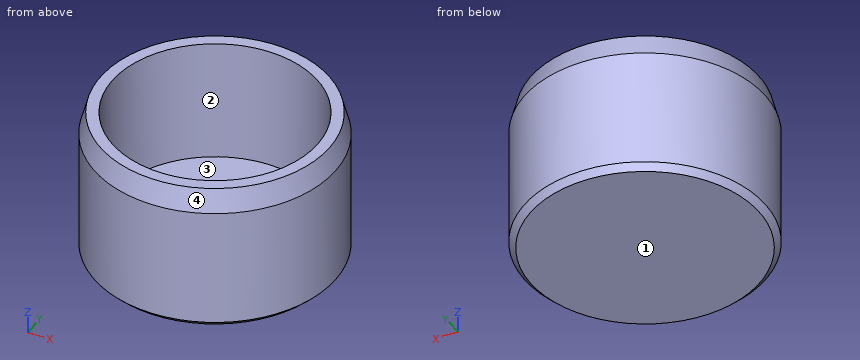
from build123d import *

# Parameters (mm, degrees)
F0_R     = 24.765
F0_R_2   = 21.082
F1_DEPTH = 30.48
F2_DEPTH = 5.08
F3_SIZE2 = 4.7397045256
F3_SIZE  = 1.27
F4_SIZE  = 1.27


with BuildPart() as f1:
    # F0 (on Top) → F1 (new body)
    with BuildSketch(Plane.XY):
        Circle(F0_R)
        Circle(F0_R_2, mode=Mode.SUBTRACT)
    extrude(amount=F1_DEPTH)

    # F0 (on Top) → F2 (join)
    with BuildSketch(Plane.XY):
        Circle(F0_R)
        Circle(F0_R_2, mode=Mode.SUBTRACT)
        Circle(F0_R_2)
    extrude(amount=F2_DEPTH)

    # F3
    f3_edges = [f1.edges().sort_by_distance(p)[0] for p in [
        (-24.765, 0, 30.48),
    ]]
    f3_side = f1.faces().sort_by_distance((-24.06454, 0, 30.48))[0]
    chamfer(f3_edges, length=F3_SIZE, length2=F3_SIZE2, reference=f3_side)

    # F4
    f4_edges = [f1.edges().sort_by_distance(p)[0] for p in [
        (-24.765, 0, 0),
    ]]
    chamfer(f4_edges, length=F4_SIZE)


solid = f1.part
Design review of the part built by this model. Coordinates are the model's own, in mm. Face numbers are marked on the shaded views. Round coordinates to 2 decimals unless told otherwise and drop trailing zeros. Write each loop counter-clockwise with the first axis right and the second up, starting at its lowest first coordinate (ties: lowest second). Pieces come first, ordered by that corner, then holes. Notation, with made-up numbers: (-19, 56.5) - (15, 56.5) arc R25 ccw to (15, 81.5) - close; hole circle Ø11 at (-31.5, 84.5). An arc over 180 degrees is marked (long way). Return JSON: item names as keys, results as strings. Group by question number.
Item 1: For probe 1 along Y at (x, z) = (0, 12.5) (3 decimals); probe 2 along Z at (x, y) = (17, -5.5); probe 3 along X at (y, z) = (0.5, 19), list the stretches that pass through material, from the lowest coordinate up. Write a range as [from, to].
Item 2: The part is to be moulded in two halves that separate along Y. For the marked faces 1, 2, 3 and 4, say which applies: pulls with the +Y half, pulls with the -Y half, needs draft (parallel to the pull), parting line crosses it, or undercut.
Item 3: We need section D-D on z = 4. Write out the cut boundary in (x, y) (3 decimals).
Item 4: We need section C-C on z = 13.5. Write out the cut boundary in (x, y) (3 decimals).
Item 5: We need section A-A on y = 0. Write out the cut boundary in (x, z) (3 decimals), and give its area (3 significant figures).
Item 6: Insertion check: P1, Ø8, axis at y = -5, z = 17.5, coming from the -X side; P2, Ø1, axis at x = -15.5, y = 12.5, coming from the +Z side; P3, Ø4, axis at y = -6, z = 3, coming from the -X side; P4, Ø5, axis at x = -8.5, y = 6.5, coming from the -Z side. Each pin has a flat end and moves straight along its axis. Give the tip position at first contact, or say it passes through.
Model answer:
{
 "1": {"probe 1": "y = [-24.765, -21.082], [21.082, 24.765]", "probe 2": "z = [0, 5.08]", "probe 3": "x = [-24.76, -21.08], [21.08, 24.76]"},
 "2": {"face 1": "needs draft", "face 2": "undercut", "face 3": "undercut", "face 4": "parting line crosses it"},
 "3": {"outline": "circle Ø49.53 at (0, 0)"},
 "4": {"outline": "circle Ø49.53 at (0, 0); hole circle Ø42.164 at (0, 0)"},
 "5": {"outline": "(-24.765, 1.27) - (-23.495, 0) - (23.495, 0) - (24.765, 1.27) - (24.765, 25.74) - (23.495, 30.48) - (21.082, 30.48) - (21.082, 5.08) - (-21.082, 5.08) - (-21.082, 30.48) - (-23.495, 30.48) - (-24.765, 25.74) - close", "area": "431 mm²"},
 "6": {"P1": "stops at x = -24.74", "P2": "stops at z = 5.08", "P3": "stops at x = -24.44", "P4": "stops at z = 0"}
}
